Design review of the part shown in the three views and the two pictorial views. Dimensions are in mm from the part's minimum x, y and z. A direction names the side the tool comes from. Round coordinates to 2 decimals unless told otherwise and drop trailing zeros. Loops run counter-clockwise (first coordinate to the right, second up) from the corner with the lowest first, then second, coordinate; pieces in that order, holes last. Notation, with made-up numbers: (-9.5, 67.25) - (-5.5, 67.25) arc R29 cw to (-5.5, 100.25) - close; hole circle Ø11 at (24.25, 50). An arc over 180 degrees is marked (long way). Return JSON: item names as keys, results as strings. Group by question number.
(1) Clearance check with flat-ended pins moving along their axes: pin 1 (6 mm diameter, centred on y = 28, z = 5, fed in from +X); pin 2 (6 mm diameter, centred on x = 15, z = 8, fed in from +Y). State where each tip first meets the part, or that it passes through.
(2) We need section A-A, the plane z = 7. Write out the cut boundary in (x, y).
(3) For the marked faces 1 and 2, list the 3-axis set-ups (+Z, -Z, +X, -X, +Y, -Y) from which the entire face can be reached by the end or side of a thin tool; tool diameter is ignored.
(4) The part is to be moulded in two halves that separate along X. For the marked faces 3, 4 and 5, say which applies: pulls with the +X half, pulls with the -X half, needs draft (parallel to the pull), parting line crosses it, or undercut.
(5) Wall thickness on L1, parallel to Y at x = 25.5, z = 1.75; L2, parallel to Y at x = 8, z = 3.5: over which ranges is each line inside the solid? List them lowest first. Write a range as [from, to].
(6) We need section B-B, the plane y = 34.5. Write out the cut boundary in (x, z), and give its area (3 significant figures).
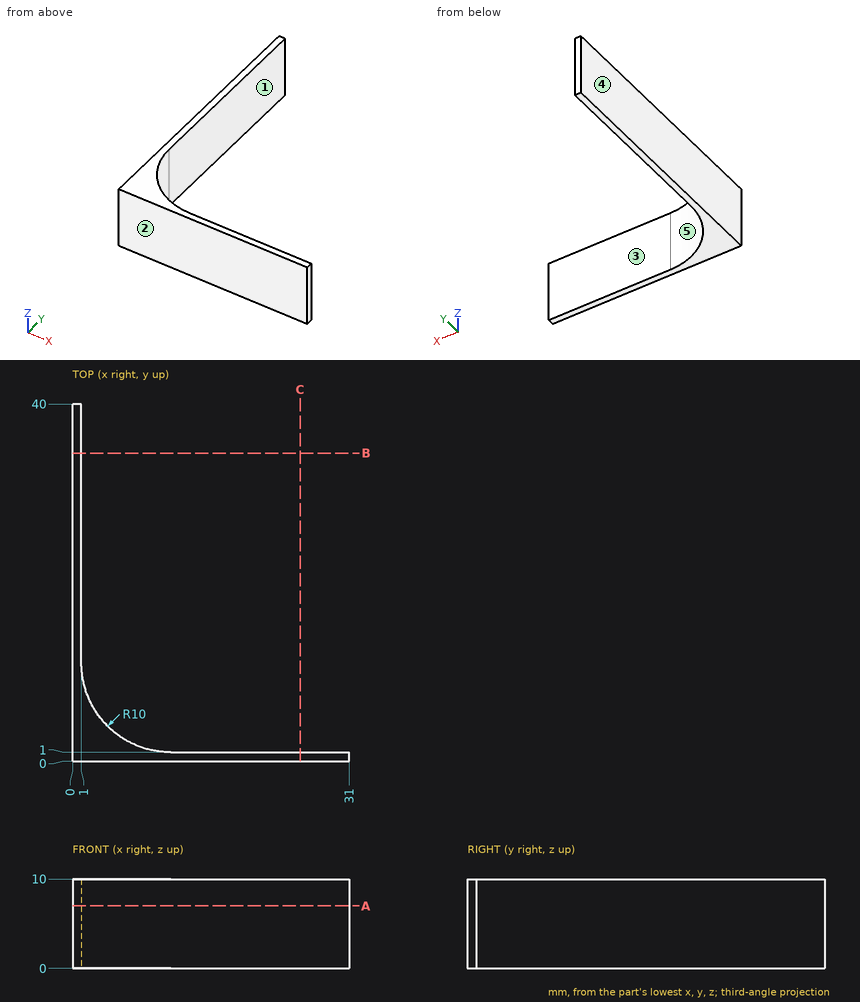
Solutions:
{
 "1": {"pin 1": "x = 1", "pin 2": "y = 1"},
 "2": {"outline": "(0, 0) - (31, 0) - (31, 1) - (11, 1) arc R10 cw to (1, 11) - (1, 40) - (0, 40) - close"},
 "3": {"face 1": "+Z, -Z, +X, +Y", "face 2": "+Z, -Z, +X, -X, -Y"},
 "4": {"face 3": "needs draft", "face 4": "pulls with the -X half", "face 5": "pulls with the +X half"},
 "5": {"L1": "[0, 1]", "L2": "[0, 1.46]"},
 "6": {"outline": "(0, 0) - (1, 0) - (1, 10) - (0, 10) - close", "area": "10.0 mm^2"}
}
